from build123d import *

# Parameters (mm, degrees)
F0_W      = 15.44
F0_H      = 8
F2_W      = 9.74
F2_H      = 8
F4_R      = 0.75
F7_DEPTH  = 100
F8_R      = 3
F9_DEPTH  = 3.5
F11_DEPTH = 7


with BuildPart() as f3:
    # F0 (on Top) → F3 section 0
    with BuildSketch(Plane.XY):
        Rectangle(F0_W, F0_H)
    # F2 (on offset) → F3 section 1
    with BuildSketch(Plane.XY.offset(12.77)):
        Rectangle(F2_W, F2_H)
    loft()

    # F4
    f4_edges = [f3.edges().sort_by_distance(p)[0] for p in [
        (4.87, 0, 12.77),
        (0, -4, 12.77),
        (-4.87, 0, 12.77),
        (0, 4, 12.77),
    ]]
    fillet(f4_edges, radius=F4_R)

    # F6 (on offset) → F7 (cut)
    with BuildSketch(Plane.YZ.offset(25)):
        with BuildLine():
            ThreePointArc((0, 7.4171952983), (1.3859292911, 7.9912660072), (1.96, 9.3771952983))
            ThreePointArc((1.96, 9.3771952983), (-1.3859292911, 10.7631245894), (0, 7.4171952983))
        make_face()
    extrude(amount=-F7_DEPTH, mode=Mode.SUBTRACT)

    # F8 (on Top) → F9 (cut)
    with BuildSketch(Plane.XY):
        with Locations((-3.8095137819, 0)):
            Circle(F8_R)
        with Locations((3.7751071386, 0)):
            Circle(F8_R)
    extrude(amount=F9_DEPTH, mode=Mode.SUBTRACT)

    # F10 (on offset) → F11 (join)
    with BuildSketch(Plane.XY.offset(12.77)):
        with BuildLine():
            ThreePointArc((0, 2.7), (-1.9091883092, -1.9091883092), (2.7, 0))
            ThreePointArc((2.7, 0), (1.9091883092, 1.9091883092), (0, 2.7))
        make_face()
    extrude(amount=F11_DEPTH)


solid = f3.part
Verification items for the finished model (mm, model axes). A direction names the side the tool comes from. Give positions to 0.01 mm unless a question says otherwise; leave off trailing zeros. Write each loop counter-clockwise with the first axis right and the second up, starting at its lowest first coordinate (ties: lowest second). Pieces come first, ordered by that corner, then holes. Notation, with made-up numbers: M -36,89.25 L 15,89.25 A26 ccw 15,103.25 Z; hole C 50,5.5 d8. An arc over 180 degrees is marked long. Put each result on its own line as item: value. Start each with the question number.
1. Go/stop test with flat-tipped pins: pin 1 Ø2 at (x, y) = (3.5, -2) entering from +Z; pin 2 Ø1 at (y, z) = (1.5, 2.5) entering from -X; pin 3 Ø2 at (y, z) = (3, 10.5) entering from +X. Record where each tip stops, or that it passes through.
2. Section check A-A (y = 1.25). Record the cut outline in (x, z), and give its area (3 significant figures).
3. Draft check along X on faces 3 (the face through (-6.34, 0.06, 6.18)), 4 (the face through (6.34, -0.06, 6.18)), 5 (the face through (3, 0, 12.77)), 6 (the face through (-0.948, 0.901, 1.726)). Enter one of: +X half, -X half, draft (parallel to the pull), parting line (faces both ways), or undercut.
4. Section check C-C (z = 18.5). Record the cut outline in (x, y).
5. Scan lines: line 1 along Z through (x, y) = (1.5, 0); line 2 along X through (y, z) = (-0.5, 2); line 3 along X through (y, z) = (-0.75, 2.75). Record each from-to range of solid material in increasing order. Write a range as [from, to].
6. Set-up check for faces 1 (the face through (0, 0, 19.77)), 2 (the face through (0.778, 0.132, 1.726)): record each of +Z, -Z, +X, -X, +Y, -Y from which the full face is reachable in a straight line by a thin tool's end or side.
7. Section check B-B (y = -0.5). Record the cut outline in (x, z).
Answer list:
1. pin 1: z = 12.77
1. pin 2: x = -7.27
1. pin 3: x = 5.6
2. outline: M -7.72,0 L -6.54,0 L -6.54,3.5 L -1.08,3.5 L -1.08,0 L 1.05,0 L 1.05,3.5 L 6.5,3.5 L 6.5,0 L 7.72,0 L 5.96,7.87 L -5.96,7.87 Z; M -5.29,10.89 L 5.29,10.89 L 5,12.18 A0.75 ccw 4.27,12.77 L 2.39,12.77 L 2.39,19.77 L -2.39,19.77 L -2.39,12.77 L -4.27,12.77 A0.75 ccw -5,12.18 Z
2. area: 122 mm2
3. face 3: -X half
3. face 4: +X half
3. face 5: draft
3. face 6: undercut
4. outline: C 0,0 d5.4
5. line 1: [3.5, 7.42], [11.34, 19.77]
5. line 2: [-7.27, -6.77], [-0.85, 0.82], [6.73, 7.27]
5. line 3: [-7.11, -6.71], [-0.9, 0.87], [6.68, 7.11]
6. face 1: +Z, +X, -X, +Y, -Y
6. face 2: -Z
7. outline: M -7.72,0 L -6.77,0 L -6.77,3.5 L -0.85,3.5 L -0.85,0 L 0.82,0 L 0.82,3.5 L 6.73,3.5 L 6.73,0 L 7.72,0 L 6.05,7.48 L -6.05,7.48 Z; M -5.2,11.27 L 5.2,11.27 L 5,12.18 A0.75 ccw 4.27,12.77 L 2.65,12.77 L 2.65,19.77 L -2.65,19.77 L -2.65,12.77 L -4.27,12.77 A0.75 ccw -5,12.18 Z
